Geometry: final body of the model. Coordinates: model frame, mm. Round coordinates to 2 decimals unless told otherwise and drop trailing zeros. Write each loop counter-clockwise with the first axis right and the second up, starting at its lowest first coordinate (ties: lowest second). Pieces come first, ordered by that corner, then holes.
from build123d import *

# Parameters (mm, degrees)
SKETCH1_W           = 176
SKETCH1_H           = 75
SKETCH1_R           = 1.6
BOSS_EXTRUDE1_DEPTH = 2
SKETCH2_W           = 72
SKETCH2_H           = 14
CUT_EXTRUDE1_DEPTH  = 2
SKETCH3_W           = 154
SKETCH3_H           = 2.5
BOSS_EXTRUDE2_DEPTH = 2
SKETCH4_W           = 2.5
SKETCH4_H           = 50
BOSS_EXTRUDE3_DEPTH = 2


with BuildPart() as part:
    # Sketch1 → Boss-Extrude1 (new body)
    with BuildSketch(Plane(origin=(0, 0, 0), x_dir=(0, 0, -1), z_dir=(1, 0, 0))):
        Rectangle(SKETCH1_W, SKETCH1_H)
        with Locations((-81, 33.5)):
            Circle(SKETCH1_R, mode=Mode.SUBTRACT)
        with Locations((81, 33.5)):
            Circle(SKETCH1_R, mode=Mode.SUBTRACT)
        with Locations((-83, -27.5)):
            Circle(SKETCH1_R, mode=Mode.SUBTRACT)
        with Locations((83, -27.5)):
            Circle(SKETCH1_R, mode=Mode.SUBTRACT)
    extrude(amount=BOSS_EXTRUDE1_DEPTH)

    # Sketch2 → Cut-Extrude1 (cut)
    with BuildSketch(Plane(origin=(2, 0, 0), x_dir=(0, 0, -1), z_dir=(1, 0, 0))):
        with Locations((0, -21.5)):
            Rectangle(SKETCH2_W, SKETCH2_H)
    extrude(amount=-CUT_EXTRUDE1_DEPTH, mode=Mode.SUBTRACT)

    # Sketch3 → Boss-Extrude2 (add)
    with BuildSketch(Plane(origin=(2, 0, 0), x_dir=(0, 0, -1), z_dir=(1, 0, 0))):
        with Locations((0, -36.25)):
            Rectangle(SKETCH3_W, SKETCH3_H)
        with Locations((0, 36.25)):
            Rectangle(SKETCH3_W, SKETCH3_H)
    extrude(amount=BOSS_EXTRUDE2_DEPTH)

    # Sketch4 → Boss-Extrude3 (add)
    with BuildSketch(Plane(origin=(2, 0, 0), x_dir=(0, 0, -1), z_dir=(1, 0, 0))):
        with Locations((-86.75, 2)):
            Rectangle(SKETCH4_W, SKETCH4_H)
        with Locations((86.75, 2)):
            Rectangle(SKETCH4_W, SKETCH4_H)
    extrude(amount=BOSS_EXTRUDE3_DEPTH)


solid = part.part
1) Section A-A on z = -9.5. Output: boundary loops of the cut face in (x, y).
2) Section D-D on z = 68. Output: boundary loops of the cut face in (x, y), plus the area to 3 significant figures.
3) Draft query along Z for faces 1 (the flat face through (2, -1, 88)), 2 (the cylindrical face through (0.99, 32.53, 82.27)), 3 (the flat face through (2, -37.5, 1)). Return one class per face: pulls with the +Z half, pulls with the -Z half, needs draft (parallel to the pull), parting line crosses it, or undercut.
4) Section C-C on y = -21. Output: boundary loops of the cut face in (x, z).
5) Line query: probe 1 along Y at (x, z) = (3.1, 53); probe 2 along Y at (x, z) = (1.05, -81); probe 3 along Z at (x, y) = (2.8, 11.5). Output: solid intervals per line, ascending.
6) Section B-B on x = 3.05. Output: boundary loops of the cut face in (y, z), plus the area to 3 significant figures.
7) First-contact query: P1, Ø3, axis at y = -27.5, z = -83, coming from the -X side; P2, Ø0.6, axis at x = 3, z = -87, coming from the +Y side; P3, Ø1.5, axis at y = -14, z = -29.5, coming from the +X side; P4, Ø1, axis at x = 3, y = -36.5, coming from the +Z side. Flat tips, straight axial feed; report the tip coordinate or a pass-through.
Filled in:
1. outline: (0, -37.5) - (4, -37.5) - (4, -35) - (2, -35) - (2, -28.5) - (0, -28.5) - close; (0, -14.5) - (2, -14.5) - (2, 35) - (4, 35) - (4, 37.5) - (0, 37.5) - close
2. outline: (0, -37.5) - (4, -37.5) - (4, -35) - (2, -35) - (2, 35) - (4, 35) - (4, 37.5) - (0, 37.5) - close
2. area: 160 mm2
3. face 1: pulls with the +Z half
3. face 2: undercut
3. face 3: needs draft
4. outline: (0, -88) - (4, -88) - (4, -85.5) - (2, -85.5) - (2, -36) - (0, -36) - close; (0, 36) - (2, 36) - (2, 85.5) - (4, 85.5) - (4, 88) - (0, 88) - close
5. probe 1: y = -37.5 to -35, 35 to 37.5
5. probe 2: y = -37.5 to 31.9, 35.1 to 37.5
5. probe 3: z = -88 to -85.5, 85.5 to 88
6. outline: (-37.5, -77) - (-35, -77) - (-35, 77) - (-37.5, 77) - close; (-23, -88) - (27, -88) - (27, -85.5) - (-23, -85.5) - close; (-23, 85.5) - (27, 85.5) - (27, 88) - (-23, 88) - close; (35, -77) - (37.5, -77) - (37.5, 77) - (35, 77) - close
6. area: 1,020 mm2
7. P1: passes through
7. P2: stops at y = 27
7. P3: stops at x = 2
7. P4: stops at z = 77
